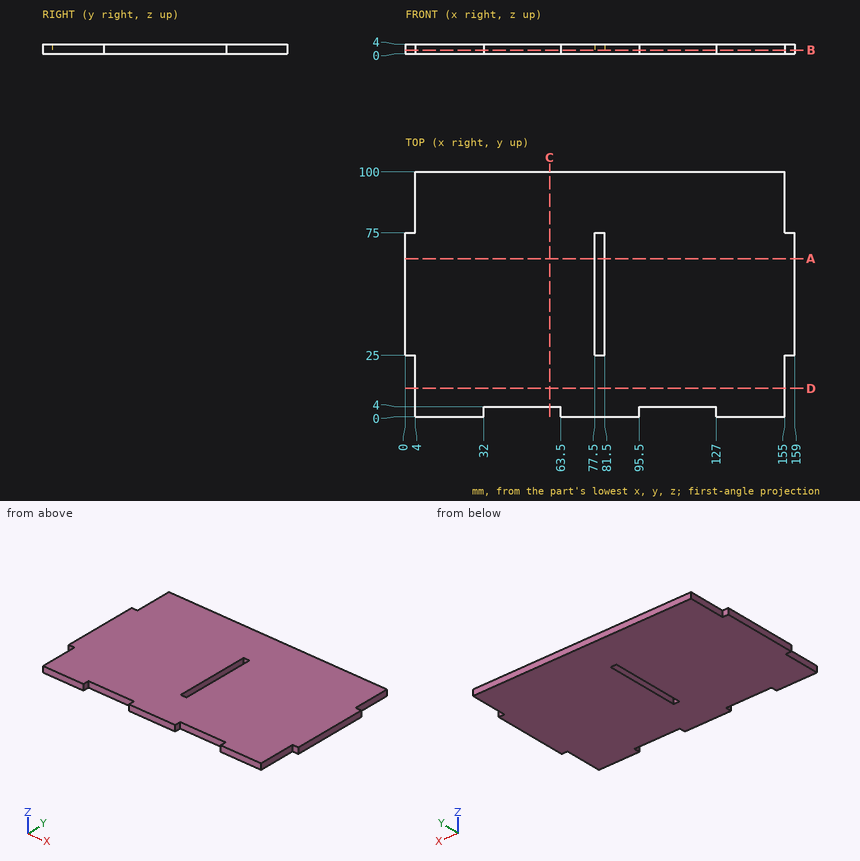
Could you check a few things on this drawing? It's one solid part, dimensions in mm from its lowest x, y, z. Coordinates: 2 decimals unless noted, no trailing zeros. Order: outer loops, then holes, each group sorted by start corner. A loop starts at its lowest first (then second) coordinate and runs counter-clockwise, first axis right, second up. Notation, with made-up numbers: (88.25, -34) - (125.25, -34) arc R16 cw to (125.25, -16) - close; hole circle Ø9 at (81.25, 53.25). An arc over 180 degrees is marked (long way). Answer as a JSON object with one key per item and string values. Group by question number.
Q1. Imagine slicing it at C-C (x = 59). Please give me the cut outline in (y, z), and give its area (3 significant figures).
Q2. Imagine slicing it at B-B (z = 1.5). Please give me the cut outline in (x, y), and give its area (3 significant figures).
Q3. Imagine slicing it at A-A (y = 64.5). Please give me the cut outline in (x, z).
Q4. I need wall thicknesses on line 1 (X direction, y = 72.5, z = 0.35); line 2 (X direction, y = 5.5, z = 0.3); line 3 (Y direction, x = 118, z = 2.75). Which ranges of each line are inside material? Lowest first, please. Write a range as from..to.
Q5. Imagine slicing it at D-D (y = 11.5). Please give me the cut outline in (x, z).
Q6. Will these pins go through, and if not, where does the flat tip stop? P1, Ø1, axis at y = 87, z = 3.5, coming from the -X side; P2, Ø2, axis at y = 2, z = 1, coming from the +X side; P3, Ø1.2, axis at x = 156.5, z = 2, coming from the +Y side.
Determined:
{
 "1": {"outline": "(4, 0) - (100, 0) - (100, 4) - (4, 4) - close", "area": "384 mm2"},
 "2": {"outline": "(0, 25) - (4, 25) - (4, 0) - (32, 0) - (32, 4) - (63.5, 4) - (63.5, 0) - (95.5, 0) - (95.5, 4) - (127, 4) - (127, 0) - (155, 0) - (155, 25) - (159, 25) - (159, 75) - (155, 75) - (155, 100) - (4, 100) - (4, 75) - (0, 75) - close; hole (77.5, 25) - (81.5, 25) - (81.5, 75) - (77.5, 75) - close", "area": "15,000 mm2"},
 "3": {"outline": "(0, 0) - (77.5, 0) - (77.5, 4) - (0, 4) - close; (81.5, 0) - (159, 0) - (159, 4) - (81.5, 4) - close"},
 "4": {"line 1": "x = 0..77.5, 81.5..159", "line 2": "x = 4..155", "line 3": "y = 4..100"},
 "5": {"outline": "(4, 0) - (155, 0) - (155, 4) - (4, 4) - close"},
 "6": {"P1": "stops at x = 4", "P2": "stops at x = 155", "P3": "stops at y = 75"}
}
